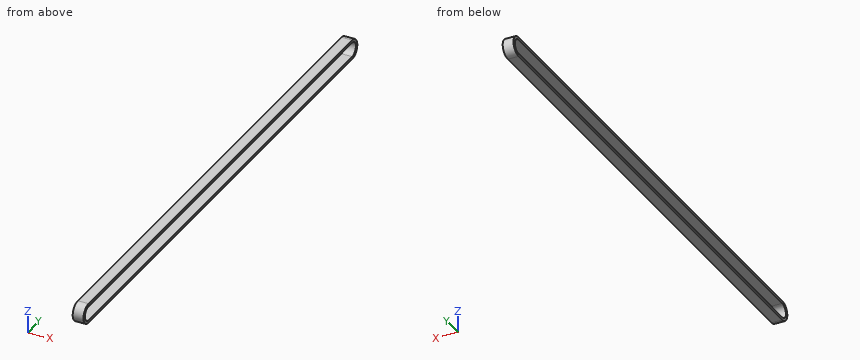
```python
from build123d import *

# Parameters (mm, degrees)
PAD_DEPTH = 3


with BuildPart() as part:
    # Sketch → Pad (new body, symmetric)
    with BuildSketch(Plane.YZ):
        with BuildLine():
            Line((-140.250008, 5.5), (143.850007, 5.5))
            ThreePointArc((143.850007, -5.5), (149.35, 0), (143.850007, 5.5))
            Line((-140.250008, -5.5), (143.850007, -5.5))
            ThreePointArc((-140.250008, 5.5), (-145.75, 0), (-140.250008, -5.5))
        make_face()
        with BuildLine():
            Line((-140.250008, 4), (143.850007, 4))
            ThreePointArc((143.850007, -4), (147.85, 0), (143.850007, 4))
            Line((-140.250008, -4), (143.850007, -4))
            ThreePointArc((-140.250008, 4), (-144.25, 0), (-140.250008, -4))
        make_face(mode=Mode.SUBTRACT)
    extrude(amount=PAD_DEPTH, both=True)


with BuildPart() as part_1:
    # Body placement: moved
    add(part.part.moved(Location((0, 0, -1.4))))


solid = part_1.part
```
The model under review builds one solid part; all positions refer to its coordinate system, in mm. Round coordinates to 2 decimals unless told otherwise and drop trailing zeros. Loops run counter-clockwise (first coordinate to the right, second up) from the corner with the lowest first, then second, coordinate; pieces in that order, holes last. Notation, with made-up numbers: (-34, -30.75) -> (-30, -30.75) arc R14 cw to (-30, -11.75) -> close; hole circle Ø6 at (51, -29.75). An arc over 180 degrees is marked (long way). Answer in a Markdown table with one row per item.
1) Consider section A-A, the plane y = -19. Write out the cut boundary in (x, z), plus the area to 3 significant figures.
Taken from the geometry:
| item | result |
|---|---|
| outline | (-3, -6.9) -> (3, -6.9) -> (3, -5.4) -> (-3, -5.4) -> close; (-3, 2.6) -> (3, 2.6) -> (3, 4.1) -> (-3, 4.1) -> close |
| area | 18.0 mm² |
2) Wall thickness on line 1 along Z through (x, y) = (0.05, -101); line 2 along Y through (x, z) = (1.6, -2); line 3 along Y through (x, z) = (-1.8, 0.5): over which ranges is each line inside the solid? List them lowest first.
Taken from the geometry:
| item | result |
|---|---|
| line 1 | z = -6.9 to -5.4, 2.6 to 4.1 |
| line 2 | y = -145.72 to -144.2, 147.8 to 149.32 |
| line 3 | y = -145.41 to -143.77, 147.37 to 149.01 |
3) For pin 1 Ø2 at (x, z) = (1, -3.5) entering from -Y, flat-tipped, find the tip position at first contact; note if it passes through.
Taken from the geometry:
| item | result |
|---|---|
| pin 1 | stops at y = -145.64 |
4) Consider section C-C, the plane x = 1.35. Write out the cut boundary in (y, z), plus the area to 3 significant figures.
Taken from the geometry:
| item | result |
|---|---|
| outline | (-140.25, -6.9) -> (143.85, -6.9) arc R5.5 ccw to (143.85, 4.1) -> (-140.25, 4.1) arc R5.5 ccw to start; hole (-140.25, -5.4) -> (143.85, -5.4) arc R4 ccw to (143.85, 2.6) -> (-140.25, 2.6) arc R4 ccw to start |
| area | 897 mm² |
5) Consider section B-B, the plane z = -1.4. Write out the cut boundary in (x, y), plus the area to 3 significant figures.
Taken from the geometry:
| item | result |
|---|---|
| outline | (-3, -145.75) -> (3, -145.75) -> (3, -144.25) -> (-3, -144.25) -> close; (-3, 147.85) -> (3, 147.85) -> (3, 149.35) -> (-3, 149.35) -> close |
| area | 18.0 mm² |
